The model under review builds one solid part; all positions refer to its coordinate system, in mm. Face numbers are marked on the shaded views. A direction names the side the tool comes from. Round coordinates to 2 decimals unless told otherwise and drop trailing zeros. Order: outer loops, then holes, each group sorted by start corner. A loop starts at its lowest first (then second) coordinate and runs counter-clockwise, first axis right, second up. Notation, with made-up numbers: M 0,37.5 L 15,37.5 A5 cw 15,43.5 Z; hole C 62.5,-21.5 d9. An arc over 180 degrees is marked long. Answer as a JSON object with one key per item and string values. Group by question number.
1. Add section C-C on x = 1. State the section outline as (y, z) points.
2. Add section D-D on z = 5.25. State the section outline as (x, y) points, and give its area (3 significant figures).
3. To check wall thickness, follow probe 1 along Z at (x, y) = (-9.25, 3.5); probe 2 along X at (y, z) = (6, 3.75); probe 3 along Y at (x, z) = (-16.25, -8.25). State the ranges of each line that lie inside material, in increasing order. Write a range as [from, to].
4. Mouldability with a two-part tool opening along X and no side actions: class the marked faces 1, 2 and 3 as released by +X, released by -X, zero draft, split by the parting line, or undercut.
5. Add section B-B on y = 5. State the section outline as (x, z) points.
6. Clearance check with flat-ended pins moving along their axes: P1, Ø1, axis at y = 5, z = -6, coming from the +X side; P2, Ø8, axis at x = -9, z = 4, coming from the +Y side. State where each tip first meets the part, or that it passes through.
7. Add section A-A on y = 1.25. State the section outline as (x, z) points.
8. Machinability: for the marked faces 4 and 5, which of the approach directions +Z, -Z, +X, -X, +Y, -Y give a long, thin tool a straight path to every point of the face, cutting with its end or side? Answer none if there is none.
```python
from build123d import *

# Parameters (mm, degrees)
ESQUISSE1_W             = 29
ESQUISSE1_H             = 27
ESQUISSE1_W_2           = 28
ESQUISSE1_H_2           = 26
ESQUISSE1_W_3           = 0.5
ESQUISSE1_H_3           = 7
BOSS_EXTRU_1_DEPTH      = 1
BOSS_EXTRU_2_DEPTH      = 7.5
ESQUISSE1_4_W           = 0.5
ESQUISSE1_4_H           = 7
BOSS_EXTRU_3_DEPTH      = 7.5
ESQUISSE7_R             = 3.5
ENL_V_MAT_EXTRU_1_DEPTH = 0.5
ESQUISSE6_R             = 3.5
ENL_V_MAT_EXTRU_2_DEPTH = 0.5


with BuildPart() as part:
    # Esquisse1 → Boss.-Extru.1 (new body)
    with BuildSketch(Plane(origin=(0, 0, 0), x_dir=(1, 0, 0), z_dir=(0, 1, 0))):
        with Locations((-8.325581395, -0.620930233)):
            Rectangle(ESQUISSE1_W, ESQUISSE1_H)
        with Locations((-8.325581395, -0.620930233)):
            Rectangle(ESQUISSE1_W_2, ESQUISSE1_H_2, mode=Mode.SUBTRACT)
        with Locations((-8.325581395, -0.620930233)):
            Rectangle(ESQUISSE1_W_2, ESQUISSE1_H_2)
        Polygon((-22.325581395, 4.879069767), (-22.325581395, 8.379069767), (-22.825581395, 8.379069767), (-22.825581395, 1.379069767), (-22.325581395, 1.379069767), align=None)
        Polygon((-22.325581395, 8.379069767), (-22.325581395, 12.379069767), (5.674418605, 12.379069767), (5.674418605, 6.379069767), (6.174418605, 6.379069767), (6.174418605, 12.879069767), (-22.825581395, 12.879069767), (-22.825581395, 8.379069767), align=None)
        with Locations((5.924418605, 2.879069767)):
            Rectangle(ESQUISSE1_W_3, ESQUISSE1_H_3)
    extrude(amount=-BOSS_EXTRU_1_DEPTH)

    # Esquisse1_3 → Boss.-Extru.2 (add)
    with BuildSketch(Plane(origin=(0, 0, 0), x_dir=(1, 0, 0), z_dir=(0, 1, 0))):
        Polygon((-22.325581395, 8.379069767), (-22.325581395, 12.379069767), (5.674418605, 12.379069767), (5.674418605, 6.379069767), (6.174418605, 6.379069767), (6.174418605, 12.879069767), (-22.825581395, 12.879069767), (-22.825581395, 8.379069767), align=None)
        Polygon((-22.325581395, -13.620930233), (-22.325581395, 1.379069767), (-22.825581395, 1.379069767), (-22.825581395, -14.120930233), (6.174418605, -14.120930233), (6.174418605, -0.620930233), (5.674418605, -0.620930233), (5.674418605, -13.620930233), align=None)
    extrude(amount=BOSS_EXTRU_2_DEPTH)

    # Esquisse1_4 → Boss.-Extru.3 (add)
    with BuildSketch(Plane(origin=(0, 0, 0), x_dir=(1, 0, 0), z_dir=(0, 1, 0))):
        with Locations((-22.575581395, 4.879069767)):
            Rectangle(ESQUISSE1_4_W, ESQUISSE1_4_H)
        with Locations((5.924418605, 2.879069767)):
            Rectangle(ESQUISSE1_4_W, ESQUISSE1_4_H)
    extrude(amount=BOSS_EXTRU_3_DEPTH)

    # Esquisse7 → Enl_v. mat.-Extru.1 (cut)
    with BuildSketch(Plane(origin=(6.174418605, 0, 0), x_dir=(0, 0, -1), z_dir=(1, 0, 0))):
        with Locations((6.379069767, 7.5)):
            Circle(ESQUISSE7_R)
    extrude(amount=-ENL_V_MAT_EXTRU_1_DEPTH, mode=Mode.SUBTRACT)

    # Esquisse6 → Enl_v. mat.-Extru.2 (cut)
    with BuildSketch(Plane.ZY.offset(22.825581395)):
        with Locations((-6.379069767, 7.5)):
            Circle(ESQUISSE6_R)
    extrude(amount=-ENL_V_MAT_EXTRU_2_DEPTH, mode=Mode.SUBTRACT)


solid = part.part
```
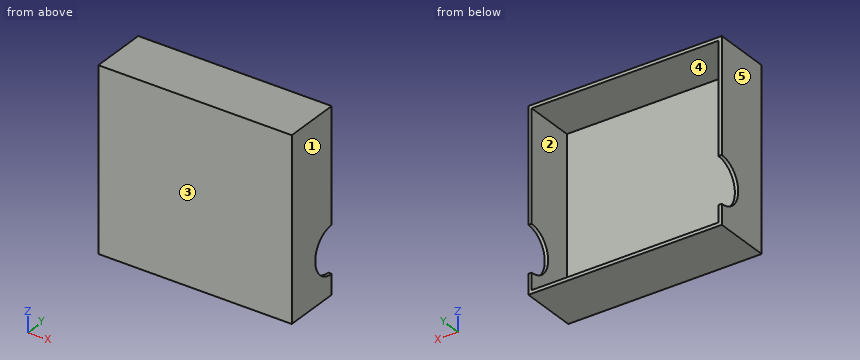
Recorded:
{
 "1": {"outline": "M -1,-12.88 L 7.5,-12.88 L 7.5,-12.38 L 0,-12.38 L 0,13.62 L 7.5,13.62 L 7.5,14.12 L -1,14.12 Z"},
 "2": {"outline": "M -22.83,-1 L 6.17,-1 L 6.17,7.5 L 5.67,7.5 L 5.67,0 L -22.33,0 L -22.33,7.5 L -22.83,7.5 Z", "area": "36.5 mm²"},
 "3": {"probe 1": "z = [-12.88, -12.38], [13.62, 14.12]", "probe 2": "x = [-22.83, -22.33], [5.67, 6.17]", "probe 3": "y = [-1, 0]"},
 "4": {"face 1": "released by +X", "face 2": "undercut", "face 3": "zero draft"},
 "5": {"outline": "M -22.83,-12.88 L 6.17,-12.88 L 6.17,-8.83 L 5.67,-8.83 L 5.67,-12.38 L -22.33,-12.38 L -22.33,-8.83 L -22.83,-8.83 Z; M -22.83,-3.93 L -22.33,-3.93 L -22.33,13.62 L 5.67,13.62 L 5.67,-3.93 L 6.17,-3.93 L 6.17,14.12 L -22.83,14.12 Z"},
 "6": {"P1": "passes through", "P2": "stops at y = 0"},
 "7": {"outline": "M -22.83,-12.88 L 6.17,-12.88 L 6.17,14.12 L -22.83,14.12 Z; hole M -22.33,-12.38 L 5.67,-12.38 L 5.67,13.62 L -22.33,13.62 Z"},
 "8": {"face 4": "+Y", "face 5": "+Z, -Z, -X, +Y, -Y"}
}
